```python
from build123d import *

# Parameters (mm, degrees)
SKETCH_W     = 166
SKETCH_H     = 10
PAD_DEPTH    = 220
SKETCH001_W  = 8.2
SKETCH001_H  = 2
POCKET_DEPTH = 220.001


with BuildPart() as part:
    # Sketch → Pad (new body)
    with BuildSketch(Plane.XY):
        with Locations((0, 5)):
            Rectangle(SKETCH_W, SKETCH_H)
    extrude(amount=PAD_DEPTH)

    # Sketch001 → Pocket (cut, through all)
    with BuildSketch(Plane.XY.offset(220)):
        with Locations((72.9, 9)):
            Rectangle(SKETCH001_W, SKETCH001_H)
        with Locations((60.9, 9)):
            Rectangle(SKETCH001_W, SKETCH001_H)
        Polygon((32.8, 10), (41, 10), (41, 8.4), (38.1, 8.4), (38.1, 2), (33.6, 2), (33.6, 8.4), (32.8, 8.4), align=None)
        with Locations((48.9, 9)):
            Rectangle(SKETCH001_W, SKETCH001_H)
        Polygon((20.8, 10), (20.8, 8.4), (21.6, 8.4), (21.6, 2), (26.1, 2), (26.1, 8.4), (29, 8.4), (29, 10), align=None)
        Polygon((17, 10), (17, 8.4), (14.1, 8.4), (14.1, 2), (9.6, 2), (9.6, 8.4), (8.8, 8.4), (8.8, 10), align=None)
    extrude(amount=-POCKET_DEPTH, mode=Mode.SUBTRACT)


solid = part.part
```
Could you check a few things on this model? Use its own coordinates, in mm. A direction names the side the tool comes from. Round coordinates to 2 decimals unless told otherwise and drop trailing zeros. Loops run counter-clockwise (first coordinate to the right, second up) from the corner with the lowest first, then second, coordinate; pieces in that order, holes last. Notation, with made-up numbers: M 10.5,-28.75 L 68.5,-28.75 A26 cw 68.5,-12.75 Z; hole C 13.25,14 d6. An arc over 180 degrees is marked long. Answer as CSV lines item,"result".
1) If I drill on probe 1 along X at (y, z) = (5.75, 129); probe 2 along Y at (x, z) = (10, 13), over which ranges is the centre line in solid material (lowest first)?
From the geometry:
probe 1,"-83 to 9.6, 14.1 to 21.6, 26.1 to 33.6, 38.1 to 83"
probe 2,"0 to 2"
2) We'd pull the mould along X, two halves only. Please class faces 1 (the flat face through (-38, 10, 108)), 2 (the flat face through (83, 5, 108)), 3 (the flat face through (26.1, 5, 112)): released by +X, released by -X, zero draft, split by the parting line, or undercut.
From the geometry:
face 1,"zero draft"
face 2,"released by +X"
face 3,"undercut"
3) For pin 1 Ø0.9 at (x, z) = (33.5, 104) entering from +Y; pin 2 Ø4 at (x, z) = (72, 91.5) entering from +Y; pin 3 Ø1.3 at (x, z) = (12.5, 62) entering from +Y, each with a flat end and sliding along its axis, tell me the tip position at first contact or that it passes through.
From the geometry:
pin 1,"y = 8.4"
pin 2,"y = 8"
pin 3,"y = 2"
4) Which directions (+Z, -Z, +X, -X, +Y, -Y) give clear straight access to the entire face, cutting with the end or side of a thin tool? Please do faces 4 (the flat face through (-1, 5, 220)), 5 (the flat face through (9.6, 5, 112)).
From the geometry:
face 4,"+Z, +X, -X, +Y, -Y"
face 5,"+Z, -Z, +Y"
5) Imagine slicing it at A-A on y = 4.25. List the corners of the cut face in (x, z) for me.
From the geometry:
outline,"M -83,0 L 9.6,0 L 9.6,220 L -83,220 Z; M 14.1,0 L 21.6,0 L 21.6,220 L 14.1,220 Z; M 26.1,0 L 33.6,0 L 33.6,220 L 26.1,220 Z; M 38.1,0 L 83,0 L 83,220 L 38.1,220 Z"
